Geometry check sheet. Reference: the model listing, model coordinates, mm. Face numbers are marked on the shaded views. A direction names the side the tool comes from. Coordinates: 2 decimals unless noted, no trailing zeros. Write each loop counter-clockwise with the first axis right and the second up, starting at its lowest first coordinate (ties: lowest second). Pieces come first, ordered by that corner, then holes. Notation, with made-up numbers: M 77,-26.75 L 135,-26.75 A24 cw 135,-13.75 Z; hole C -1,54 d5. An arc over 180 degrees is marked long. Write item = value, one per line. Start each with the question number.
```python
from build123d import *

# Parameters (mm, degrees)
BOSS_EXTRUDE1_DEPTH       = 3.175
F_4_CLEARANCE_HOLE1_D     = 2.9464
F_4_CLEARANCE_HOLE1_DEPTH = 3.302
F_4_CLEARANCE_HOLE1_TIP   = 0.885187864
CUT_EXTRUDE1_REACH        = 5.175
SKETCH4_R                 = 4.7625


with BuildPart() as part:
    # Sketch1 → Boss-Extrude1 (new body)
    with BuildSketch(Plane.XY):
        Polygon((7.9375, -3.175), (10.8966, -3.175), (10.8966, 3.175), (-10.8966, 3.175), (-10.8966, -3.175), (-7.9375, -3.175), (-7.9375, -22.225), (-10.8966, -22.225), (-10.8966, -28.575), (10.8966, -28.575), (10.8966, -22.225), (7.9375, -22.225), align=None)
    extrude(amount=BOSS_EXTRUDE1_DEPTH)

    # #4 Clearance Hole1
    with Locations(Plane.XY.offset(3.175)):
        with Locations((0, 0), (0, -25.4)):
            Hole(F_4_CLEARANCE_HOLE1_D / 2, depth=F_4_CLEARANCE_HOLE1_DEPTH)
            with Locations((0, 0, -(F_4_CLEARANCE_HOLE1_DEPTH + F_4_CLEARANCE_HOLE1_TIP / 2))):  # 118° drill point
                Cone(0, F_4_CLEARANCE_HOLE1_D / 2, F_4_CLEARANCE_HOLE1_TIP, mode=Mode.SUBTRACT)

    # Sketch4 → Cut-Extrude1 (cut, up to next)
    with BuildSketch(Plane.XY.offset(3.175), mode=Mode.PRIVATE) as cut_extrude1_sk1:
        with Locations((0, -12.7)):
            Circle(SKETCH4_R)
    cut_extrude1_tool1 = extrude(cut_extrude1_sk1.sketch, amount=-CUT_EXTRUDE1_REACH, mode=Mode.PRIVATE) & part.part
    add(cut_extrude1_tool1.solids().sort_by_distance((0, -12.7, 3.175))[0], mode=Mode.SUBTRACT)


solid = part.part
```
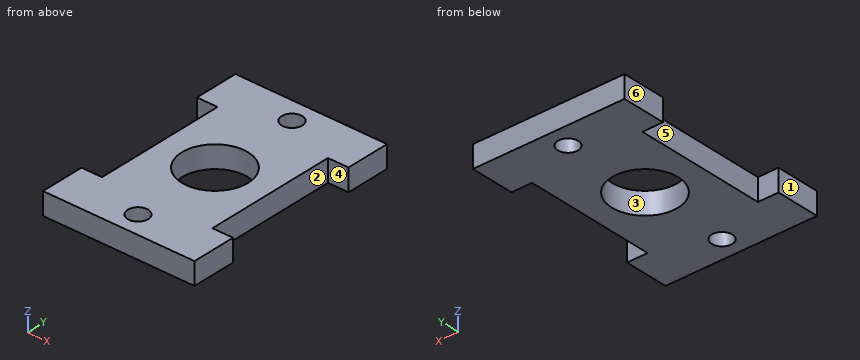
Q1. Draft check along X on the marked faces 1, 2 and 3. Enter one of: pulls with the +X half, pulls with the -X half, needs draft (parallel to the pull), parting line crosses it, or undercut.
Q2. Cross-section at D-D on x = -2.75. Enter the section's corners in (y, z) (3 decimals).
Q3. Cross-section at C-C on z = 1.65. Enter the section's corners in (x, y) (1 decimal), and give its area (3 significant figures).
Q4. Set-up check for the marked faces 4, 5 and 6: record each of +Z, -Z, +X, -X, +Y, -Y from which the full face is reachable in a straight line by a thin tool's end or side.
Q5. Cross-section at B-B on x = 0. Enter the section's corners in (y, z) (1 decimal), and give its area (3 significant figures).
Q6. Gauge pin test, flat end, axial feed: pin 1 (1 mm diameter, centred on y = -16, z = 1.5, fed in from -X). Record the tip position at first contact, or that the pin passes through.
Q7. Scan lines: L1, parallel to Y at x = 0, z = 2.15 (1 decimal); L2, parallel to Y at x = -2, z = 0.9 (3 decimals); L3, parallel to X at y = -20, z = 1.1. Record each from-to range of solid material in increasing order.
Q8. Cross-section at A-A on y = 0. Enter the section's corners in (x, z) (3 decimals).
Values found:
q1.face_1 = pulls with the -X half
q1.face_2 = pulls with the +X half
q1.face_3 = undercut
q2.outline = M -28.575,0 L -16.588,0 L -16.588,3.175 L -28.575,3.175 Z; M -8.812,0 L 3.175,0 L 3.175,3.175 L -8.812,3.175 Z
q3.outline = M -10.9,-28.6 L 10.9,-28.6 L 10.9,-22.2 L 7.9,-22.2 L 7.9,-3.2 L 10.9,-3.2 L 10.9,3.2 L -10.9,3.2 L -10.9,-3.2 L -7.9,-3.2 L -7.9,-22.2 L -10.9,-22.2 Z; hole C 0,-12.7 d9.5; hole C 0,-25.4 d2.9; hole C 0,0 d2.9
q3.area = 494 mm²
q4.face_4 = +Z, -Z, +X
q4.face_5 = +Z, -Z, -X
q4.face_6 = +Z, -Z, -X, +Y, -Y
q5.outline = M -28.6,0 L -26.9,0 L -26.9,3.2 L -28.6,3.2 Z; M -23.9,0 L -17.5,0 L -17.5,3.2 L -23.9,3.2 Z; M -7.9,0 L -1.5,0 L -1.5,3.2 L -7.9,3.2 Z; M 1.5,0 L 3.2,0 L 3.2,3.2 L 1.5,3.2 Z
q5.area = 51.9 mm²
q6.pin_1 = -7.94
q7.L1 = -28.6 to -26.9, -23.9 to -17.5, -7.9 to -1.5, 1.5 to 3.2
q7.L2 = -28.575 to -17.022, -8.378 to 3.175
q7.L3 = -7.94 to 7.94
q8.outline = M -10.897,0 L -1.473,0 L -1.473,3.175 L -10.897,3.175 Z; M 1.473,0 L 10.897,0 L 10.897,3.175 L 1.473,3.175 Z
